Geometry check sheet. Reference: the model listing, model coordinates, mm. Coordinates: 2 decimals unless noted, no trailing zeros. Loops run counter-clockwise (first coordinate to the right, second up) from the corner with the lowest first, then second, coordinate; pieces in that order, holes last.
from build123d import *

# Parameters (mm, degrees)
SKETCH1_R           = 14.2875
BOSS_EXTRUDE1_DEPTH = 1.27


with BuildPart() as part:
    # Sketch1 → Boss-Extrude1 (new body, symmetric)
    with BuildSketch(Plane(origin=(0, 0, 0), x_dir=(0, 0, -1), z_dir=(1, 0, 0))):
        Polygon((-201.134911254, -254), (-201.134911254, 123.825), (297.346438746, 123.825), (322.746438746, 123.825), (322.746438746, 47.625), (297.346438746, 47.625), (297.346438746, -177.8), (322.746438746, -177.8), (322.746438746, -254), (297.346438746, -254), (246.546438746, -254), (246.546438746, 73.025), (-150.334911254, 73.025), (-150.334911254, -254), align=None)
        with Locations((-175.734911254, 98.425)):
            Circle(SKETCH1_R, mode=Mode.SUBTRACT)
    extrude(amount=BOSS_EXTRUDE1_DEPTH, both=True)


solid = part.part
(1) Sectioned sample at D-D on z = 106. Record the cut outline in (x, y) (3 decimals).
Findings:
outline: (-1.27, 73.025) - (1.27, 73.025) - (1.27, 123.825) - (-1.27, 123.825) - close
(2) Sectioned sample at A-A on y = -47.5. Record the cut outline in (x, z), and give its area (3 significant figures).
Findings:
outline: (-1.27, -297.35) - (1.27, -297.35) - (1.27, -246.55) - (-1.27, -246.55) - close; (-1.27, 150.33) - (1.27, 150.33) - (1.27, 201.13) - (-1.27, 201.13) - close
area: 258 mm2
(3) Sectioned sample at B-B on x = -0.65. Record the cut outline in (y, z) (1 decimal), and give its area (3 significant figures).
Findings:
outline: (-254, -322.7) - (-177.8, -322.7) - (-177.8, -297.3) - (47.6, -297.3) - (47.6, -322.7) - (123.8, -322.7) - (123.8, 201.1) - (-254, 201.1) - (-254, 150.3) - (73, 150.3) - (73, -246.5) - (-254, -246.5) - close; hole circle Ø28.6 at (98.4, 175.7)
area: 61,800 mm2
(4) Scan lines: L1, parallel to Z at x = 0.85, y = -226; L2, parallel to Z at x = 1, y = -29; L3, parallel to Y at x = -0.8, z = 81.5 (3 decimals). Record each from-to range of solid material in increasing order.
Findings:
L1: z = -322.75 to -246.55, 150.33 to 201.13
L2: z = -297.35 to -246.55, 150.33 to 201.13
L3: y = 73.025 to 123.825
(5) Sectioned sample at C-C on y = -229. Record the cut outline in (x, z), and give its area (3 significant figures).
Findings:
outline: (-1.27, -322.75) - (1.27, -322.75) - (1.27, -246.55) - (-1.27, -246.55) - close; (-1.27, 150.33) - (1.27, 150.33) - (1.27, 201.13) - (-1.27, 201.13) - close
area: 323 mm2
(6) Gauge pin test, flat end, axial feed: pin 1 Ø0.8 at (x, y) = (0, -101) entering from -Z. Record the tip position at first contact, or that the pin passes through.
Findings:
pin 1: stops at z = -297.35
(7) Draft check along Z on faces 1 (the flat face through (-1.27, 76, -43)), 2 (the cylindrical face through (-0.02, 89.73, 187.07)). Enter one of: +Z half, -Z half, draft (parallel to the pull), parting line (faces both ways), or undercut.
Findings:
face 1: draft
face 2: undercut
